Could you check a few things on this model? Use its own coordinates, in mm. A direction names the side the tool comes from. Round coordinates to 2 decimals unless told otherwise and drop trailing zeros. Write each loop counter-clockwise with the first axis right and the second up, starting at its lowest first coordinate (ties: lowest second). Pieces come first, ordered by that corner, then holes. Notation, with made-up numbers: (69.5, 72) -> (80.5, 72) arc R29 cw to (80.5, 103) -> close; hole circle Ø4 at (-28.5, 46.5). An arc over 180 degrees is marked (long way). Answer in a Markdown table with one row per item. Add a question column.
```python
from build123d import *

# Parameters (mm, degrees)
F0_R     = 12.7
F0_R_2   = 10.9982
F1_DEPTH = 5.715
F0_R_3   = 9.7155
F2_DEPTH = 15.24
F3_R     = 0.762


with BuildPart() as f1:
    # F0 (on Top) → F1 (new body)
    with BuildSketch(Plane.XY):
        Circle(F0_R)
        Circle(F0_R_2, mode=Mode.SUBTRACT)
    extrude(amount=F1_DEPTH)

    # F0 (on Top) → F2 (join)
    with BuildSketch(Plane.XY):
        Circle(F0_R)
        Circle(F0_R_2, mode=Mode.SUBTRACT)
        Circle(F0_R_2)
        Circle(F0_R_3, mode=Mode.SUBTRACT)
    extrude(amount=-F2_DEPTH)

    # F3
    f3_edges = [f1.edges().sort_by_distance(p)[0] for p in [
        (-9.7155, 0, -15.24),
        (-12.7, 0, -15.24),
        (-12.7, 0, 5.715),
        (-10.9982, 0, 5.715),
    ]]
    fillet(f3_edges, radius=F3_R)


solid = f1.part
```
(1) On a 3-axis mill with a long thin cutter (end or side, diameter ignored), from which of +Z, -Z, +X, -X, +Y, -Y can I reach the whole of each face in a straight line? I mean faces 4 (the face through (0, -10, 0)), 5 (the face through (-2.106, -9.484, -7.138)). Say none if no direction works.
(2) I need wall thicknesses on L1, parallel to Y at x = 0, z = 1.7; L2, parallel to Y at x = 0, z = -7.75; L3, parallel to X at y = -0.25, z = -13.75. Which ranges of each line are inside material? Lowest first, please.
(3) If we mould it in two halves opening along Y, with no side actions, what happens to faces 1 (the face through (-2.75, -12.4, -4.63)), 2 (the face through (-8.73, -6.69, 2.44)), 3 (the face through (0, -11, -15.24))? For each: pulls with the +Y half, pulls with the -Y half, needs draft (parallel to the pull), parting line crosses it, or undercut.
(4) Suppose I cut it at C-C, the plane z = -7. Please give me the cut outline in (x, y).
(5) For P1, Ø4, axis at x = -5.5, z = -7, coming from the +Y side; P2, Ø6.5, axis at x = 3.5, y = -5.5, coming from the +Z side; P3, Ø5, axis at x = -7, z = -2.5, coming from the +Y side, each with a flat end and sliding along its axis, tell me the tip position at first contact or that it passes through.
Response:
| question | item | result |
|---|---|---|
| 1 | face 4 | +Z |
| 1 | face 5 | +Z, -Z |
| 2 | L1 | -12.7 to -11, 11 to 12.7 |
| 2 | L2 | -12.7 to -9.72, 9.72 to 12.7 |
| 2 | L3 | -12.7 to -9.71, 9.71 to 12.7 |
| 3 | face 1 | parting line crosses it |
| 3 | face 2 | undercut |
| 3 | face 3 | needs draft |
| 4 | outline | circle Ø25.4 at (0, 0); hole circle Ø19.43 at (0, 0) |
| 5 | P1 | y = 12.21 |
| 5 | P2 | z = 0 |
| 5 | P3 | y = 11.88 |
